Autodesk Inventor part; units mm, degrees
ref_plane "YZ Plane" through (0, 0, 0) normal (1, 0, 0) x (0, 1, 0)
ref_plane "XZ Plane" through (0, 0, 0) normal (0, 1, 0) x (-1, 0, 0)
ref_plane "XY Plane" through (0, 0, 0) normal (0, 0, 1) x (1, 0, 0)
sketch "Sketch1" plane through (0, 0, 0) normal (0, 0, 1) x (1, 0, 0)
  circle A0 centre (-3.3222, -5.7216) radius 11.7
  circle A1 centre (-3.3222, -5.7216) radius 12.7
  point P0 (0, 0)
  dimension "d3" = 1
  dimension "d4" = 25.4
extrude "Extrusion1" add sketch "Sketch1" against normal blind 3
sketch "Sketch3" plane through (-3.3222, -5.7216, 0) normal (0, 0, 1) x (1, 0, 0)
  circle A0 centre (0, 0) radius 11.7
  circle A1 centre (0, 0) radius 12.7
  circle A2 centre (0, 0) radius 11.5
  circle A3 centre (0, 0) radius 14.9
  point P0 (3.3222, 5.7216)
  dimension "d12" = 23
  dimension "d14" = 29.8
extrude "Extrusion3" add sketch "Sketch3" along normal blind 1 contours A0 | A1 | A3
sketch "Sketch4" plane through (-3.3222, -5.7216, 1) normal (0, 0, 1) x (1, 0, 0)
  circle A0 centre (0, 0) radius 14.9
  circle A1 centre (0, 0) radius 12.6
  circle A2 centre (0, 0) radius 13.6
  point P0 (3.3222, 5.7216)
  dimension "d17" = 1
  dimension "d19" = 25.2
extrude "Extrusion4" add sketch "Sketch4" along normal blind 3 contours A2
properties part number "Eyepiece tube filter holder"
CAD build for the part. Positions are in the model's coordinates, mm. A direction names the side the tool comes from. Round coordinates to 2 decimals unless told otherwise and drop trailing zeros. Loops run counter-clockwise (first coordinate to the right, second up) from the corner with the lowest first, then second, coordinate; pieces in that order, holes last.
(1) Drop flat-ended pins along their axis: pin 1 (1.5 mm diameter, centred on y = -10.5, z = -2, fed in from -X); pin 2 (3 mm diameter, centred on x = -1.5, z = 0, fed in from +Y). Give the stop position or say it passes through.
(2) Cut at A-A (y = -1.25). Give the cut face in (x, z).
(3) Cut at B-B (x = 4). Give the cut face in (y, z), plus the area to 3 significant figures.
(4) Cut at C-C (x = 8.75). Give the cut face in (y, z).
(5) Cut at D-D (z = 0.5). Give the cut face in (x, y), plus the area to 3 significant figures.
(6) Which spindle directions (+Z, -Z, +X, -X, +Y, -Y) get a long thin tool onto all of the face, cutting with end or side? Do faces 4 (the cylindrical face through (-16.91, -6.32, 2.48)), 5 (the cylindrical face through (7.486, -10.203, -1.479)), 6 (the cylindrical face through (-5.262, -20.495, 0.493)). Say none if no direction does.
(7) Two-plate mould, pull along X, no slides. Class faces 1 (the flat face through (8, -9, 1)), 2 (the flat face through (8, 1, 0)), 3 (the cylindrical face through (-6.08, -18.12, -1.48)): +X half, -X half, draft (parallel to the pull), parting line (faces both ways), or undercut.
(8) Wall check: line 1 along Y through (x, z) = (6.5, 0.5); line 2 along X through (y, z) = (-7.5, -1.25); line 3 along X through (y, z) = (-8.5, 1.75). Give the ranges that are in metal, low to high.
Findings below:
1. pin 1: stops at x = -15.37
1. pin 2: stops at y = 9.17
2. outline: (-17.54, 0) - (-15.21, 0) - (-15.21, -3) - (-14.13, -3) - (-14.13, 0) - (-13.92, 0) - (-13.92, 1) - (-15.1, 1) - (-15.1, 4) - (-16.17, 4) - (-16.17, 1) - (-17.54, 1) - close; (7.27, 0) - (7.49, 0) - (7.49, -3) - (8.56, -3) - (8.56, 0) - (10.89, 0) - (10.89, 1) - (9.52, 1) - (9.52, 4) - (8.46, 4) - (8.46, 1) - (7.27, 1) - close
3. outline: (-18.7, 0) - (-16.1, 0) - (-16.1, -3) - (-14.85, -3) - (-14.85, 0) - (-14.59, 0) - (-14.59, 1) - (-15.98, 1) - (-15.98, 4) - (-17.18, 4) - (-17.18, 1) - (-18.7, 1) - close; (3.15, 0) - (3.4, 0) - (3.4, -3) - (4.66, -3) - (4.66, 0) - (7.26, 0) - (7.26, 1) - (5.74, 1) - (5.74, 4) - (4.53, 4) - (4.53, 1) - (3.15, 1) - close
3. area: 23.0 mm2
4. outline: (-14.45, 0) - (-9.67, 0) - (-9.67, -3) - (-1.78, -3) - (-1.78, 0) - (3.01, 0) - (3.01, 1) - (0.54, 1) - (0.54, 4) - (-2.11, 4) - (-2.11, 1) - (-9.33, 1) - (-9.33, 4) - (-11.98, 4) - (-11.98, 1) - (-14.45, 1) - close
5. outline: circle Ø29.8 at (-3.32, -5.72); hole circle Ø23 at (-3.32, -5.72)
5. area: 282 mm2
6. face 4: +Z
6. face 5: -Z
6. face 6: +Z, -Z
7. face 1: undercut
7. face 2: draft
7. face 3: parting line
8. line 1: y = -16.93 to -11.7, 0.26 to 5.48
8. line 2: x = -15.9 to -14.89, 8.24 to 9.25
8. line 3: x = -16.64 to -15.61, 8.97 to 9.99
